Autodesk Inventor part; units mm, degrees
ref_plane "YZ Plane" through (0, 0, 0) normal (1, 0, 0) x (0, 1, 0)
ref_plane "XZ Plane" through (0, 0, 0) normal (0, 1, 0) x (-1, 0, 0)
ref_plane "XY Plane" through (0, 0, 0) normal (0, 0, 1) x (1, 0, 0)
sketch "スケッチ1" plane through (0, 0, 0) normal (0, 0, 1) x (1, 0, 0)
  line L0 (-25, 12.5) -> (25, 12.5)
  line L1 (25, 12.5) -> (25, -12.5)
  line L2 (25, -12.5) -> (-25, -12.5)
  line L3 (-25, -12.5) -> (-25, 12.5)
  line L4 (-23, 10.5) -> (23, 10.5)
  line L5 (23, 10.5) -> (23, -10.5)
  line L6 (23, -10.5) -> (-23, -10.5)
  line L7 (-23, -10.5) -> (-23, 10.5)
  point P0 (0, 0)
  dimension "d0" = 50
  dimension "d1" = 25
  dimension "d2" = 12.5
  dimension "d3" = 25
  dimension "d4" = 2
  dimension "d5" = 2
  dimension "d6" = 2
  dimension "d7" = 2
extrude "押し出し1" add sketch "スケッチ1" along normal blind 25
sketch "スケッチ4" plane through (-25, -12.5, 0) normal (0, -1, 0) x (1, 0, 0)
  line L0 (50, 25) -> (0, 25)
  line L1 (0, 0) -> (0, 25)
  line L2 (50, 0) -> (0, 0)
  line L3 (50, 0) -> (50, 25)
  point P0 (25, 0)
  point P1 (5, 20)
  point P2 (5, 5)
  point P3 (45, 5)
  point P4 (45, 20)
  dimension "d27" = 5
  dimension "d28" = 5
  dimension "d29" = 5
  dimension "d30" = 5
  dimension "d31" = 5
  dimension "d32" = 5
  dimension "d33" = 5
  dimension "d34" = 5
hole "Hole3" at (-20, -12.5, 20) at (-20, -12.5, 5) at (20, -12.5, 5) at (20, -12.5, 20) direction (0, 1, 0) diameter 2.459 end up to surface
sketch "スケッチ5" plane through (-25, 12.5, 0) normal (0, 1, 0) x (1, 0, 0)
  line L0 (0, 0) -> (50, 0)
  line L1 (0, 0) -> (0, -25)
  point P0 (25, 0)
  point P1 (10, -12.5)
  point P2 (30, -12.5)
  dimension "d42" = 10
  dimension "d43" = 20
  dimension "d44" = 12.5
  dimension "d45" = 12.5
hole "Hole4" at (-15, 12.5, 12.5) at (5, 12.5, 12.5) direction (0, -1, 0) diameter 6 end up to surface
equation "\"d5\" = d4"
equation "\"d6\" = d4"
equation "\"d7\" = d4"
properties part number "JointC0"
Work out the finished part from the listing and answer in its coordinate system (mm). A direction names the side the tool comes from. Give positions to 0.01 mm unless a question says otherwise; leave off trailing zeros. Write each loop counter-clockwise with the first axis right and the second up, starting at its lowest first coordinate (ties: lowest second). Pieces come first, ordered by that corner, then holes. Notation, with made-up numbers: (-9.5, -1) - (-5.5, -1) arc R38 ccw to (-5.5, 38) - close; hole circle Ø9 at (-6.75, 16). An arc over 180 degrees is marked (long way). One line per item, written item: value. Start each with the question number.
1. Given pin 1 (2 mm diameter, centred on x = 20, z = 5, fed in from -Y), flat-ended and moving along its own axis, determine where the tip first touches the part or whether it passes through.
2. Find section B-B (x = -7.5). Write down the section's boundary in (y, z), then the cut area to 3 significant figures.
3. Consider probe 1 along X at (y, z) = (11.8, 12.5); probe 2 along X at (y, z) = (-10.85, 5); probe 3 along Z at (x, y) = (20, -11). Determine where each line is inside the solid, lowest interval first.
4. Find section C-C (y = -1.5). Write down the section's boundary in (x, z), then the cut area to 3 significant figures.
5. For faces 1 (the cylindrical face through (2.97, 11.49, 10.29)), 2 (the flat face through (0, 10.5, 12)), 3 (the cylindrical face through (20.471, -11.486, 18.864)), determine the directions among +Z, -Z, +X, -X, +Y, -Y from which every point of the face is accessible in a straight line to the end or side of a thin tool.
6. Find section D-D (x = -15). Write down the section's boundary in (y, z).
7. For a pull along Y with two mould halves and no side action, classify faces 4 (the flat face through (-2, -11, 0)), 5 (the flat face through (23, 0, 12)), 6 (the flat face through (0, -10.5, 12)), 7 (the flat face through (0, 12.5, 12)) as +Y half, -Y half, draft (parallel to the pull), parting line (faces both ways), or undercut.
8. Find section A-A (z = 12.5). Write down the section's boundary in (x, y), then the cut area to 3 significant figures.
Geometry results:
1. pin 1: y = 10.5
2. outline: (-12.5, 0) - (-10.5, 0) - (-10.5, 25) - (-12.5, 25) - close; (10.5, 0) - (12.5, 0) - (12.5, 25) - (10.5, 25) - close
2. area: 100 mm2
3. probe 1: -25 to -18, -12 to 2, 8 to 25
3. probe 2: -25 to -21.23, -18.77 to 18.77, 21.23 to 25
3. probe 3: 0 to 3.77, 6.23 to 18.77, 21.23 to 25
4. outline: (-25, 0) - (-23, 0) - (-23, 25) - (-25, 25) - close; (23, 0) - (25, 0) - (25, 25) - (23, 25) - close
4. area: 100 mm2
5. face 1: +Y
5. face 2: +Z, -Z
5. face 3: -Y
6. outline: (-12.5, 0) - (-10.5, 0) - (-10.5, 25) - (-12.5, 25) - close; (10.5, 0) - (12.5, 0) - (12.5, 9.5) - (10.5, 9.5) - close; (10.5, 15.5) - (12.5, 15.5) - (12.5, 25) - (10.5, 25) - close
7. face 4: draft
7. face 5: undercut
7. face 6: undercut
7. face 7: +Y half
8. outline: (-25, -12.5) - (25, -12.5) - (25, 12.5) - (8, 12.5) - (8, 10.5) - (23, 10.5) - (23, -10.5) - (-23, -10.5) - (-23, 10.5) - (-18, 10.5) - (-18, 12.5) - (-25, 12.5) - close; (-12, 10.5) - (2, 10.5) - (2, 12.5) - (-12, 12.5) - close
8. area: 260 mm2
